```python
from build123d import *

# Parameters (mm, degrees)
SKETCH1_R           = 3.6
BOSS_EXTRUDE1_DEPTH = 14
BOSS_EXTRUDE2_DEPTH = 1.5
BOSS_EXTRUDE3_DEPTH = 9
CIRPATTERN1_COUNT   = 2


with BuildPart() as part:
    # Sketch1 → Boss-Extrude1 (new body)
    with BuildSketch(Plane(origin=(0, 0, 0), x_dir=(0, 0, -1), z_dir=(1, 0, 0))):
        Circle(SKETCH1_R)
    extrude(amount=BOSS_EXTRUDE1_DEPTH)

    # Sketch2 → Boss-Extrude2 (add)
    with BuildSketch(Plane.ZY):
        Polygon((-5, 16.642259954), (-3.505186232, 16.766886588), (-2.117676372, 0.124626634), (-3.61249014, 0), align=None)
    boss_extrude2 = extrude(amount=-BOSS_EXTRUDE2_DEPTH)

    # Sketch4 → Boss-Extrude3 (add)
    with BuildSketch(Plane(origin=(1.5, 0, 0), x_dir=(0, 0, -1), z_dir=(1, 0, 0))):
        Polygon((5, 16.642259954), (3.505186232, 16.766886588), (3.380559598, 15.27207282), (4.875373366, 15.147446186), align=None)
    boss_extrude3 = extrude(amount=BOSS_EXTRUDE3_DEPTH)

    # CirPattern1: Boss-Extrude2, Boss-Extrude3 ×2 about axis
    cirpattern1_axis = Axis((7, 0, 0), (0, 1, 0))
    add([boss_extrude2.rotate(cirpattern1_axis, i * 360 / CIRPATTERN1_COUNT) for i in range(1, CIRPATTERN1_COUNT)])
    add([boss_extrude3.rotate(cirpattern1_axis, i * 360 / CIRPATTERN1_COUNT) for i in range(1, CIRPATTERN1_COUNT)])


solid = part.part
```
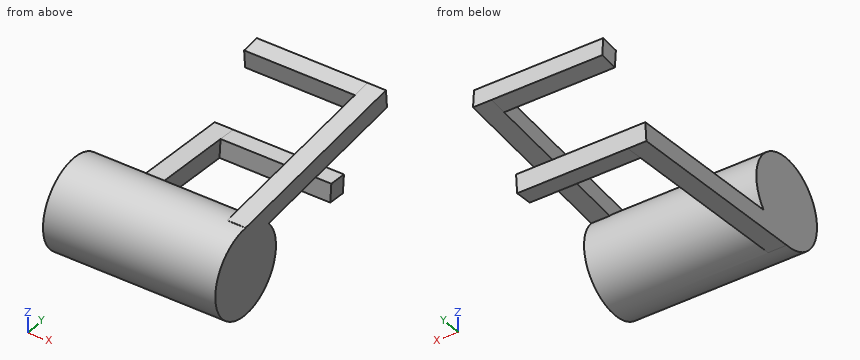
Geometry check sheet. Reference: the model listing, model coordinates, mm. Coordinates: 2 decimals unless noted, no trailing zeros. Write each loop counter-clockwise with the first axis right and the second up, starting at its lowest first coordinate (ties: lowest second). Pieces come first, ordered by that corner, then holes. Notation, with made-up numbers: M 16.5,83 L 44.5,83 A30 cw 44.5,107 Z; hole C 71,65 d5. An arc over 180 degrees is marked long. Use one line per item in the form item = value. Start each with the question number.
1) Thickness scan on probe 1 along Z at (x, y) = (2.5, 0); probe 2 along Z at (x, y) = (7.5, -2.5); probe 3 along Y at (x, z) = (9, 4.5). Record the ranges inside material, lowest first. Write a range as from..to.
2) Go/stop test with flat-tipped pins: pin 1 Ø3 at (y, z) = (7.5, -3.5) entering from +X; pin 2 Ø1.3 at (y, z) = (9.5, 4) entering from -X; pin 3 Ø4 at (x, y) = (5.5, 3.5) entering from +Z. Record where each tip stops, or that it passes through.
3) Section check D-D on y = 1.75. Enter the section's corners in (x, z), and give its area (3 significant figures).
4) Section check B-B on y = 9.75. Enter the section's corners in (x, z), and give its area (3 significant figures).
5) Section check C-C on x = 2.25. Enter the section's corners in (y, z), and give its area (3 significant figures).
6) Section check A-A on x = 8.5. Enter the section's corners in (y, z), and give its area (3 significant figures).
Responses:
q1.probe_1 = -3.6..3.6
q1.probe_2 = -2.59..2.59
q1.probe_3 = 15.18..16.68
q2.pin_1 = 1.5
q2.pin_2 = 12.5
q2.pin_3 = 3.27
q3.outline = M 0,-3.76 L 1.5,-3.76 L 1.5,-3.15 L 14,-3.15 L 14,3.76 L 12.5,3.76 L 12.5,3.15 L 0,3.15 Z
q3.area = 89.9 mm2
q4.outline = M 0,-4.43 L 1.5,-4.43 L 1.5,-2.92 L 0,-2.92 Z; M 12.5,2.92 L 14,2.92 L 14,4.43 L 12.5,4.43 Z
q4.area = 4.52 mm2
q5.outline = C 0,0 d7.2; M 15.15,-4.88 L 16.64,-5 L 16.77,-3.51 L 15.27,-3.38 Z
q5.area = 43.0 mm2
q6.outline = C 0,0 d7.2; M 15.15,-4.88 L 16.64,-5 L 16.77,-3.51 L 15.27,-3.38 Z; M 15.15,4.88 L 15.27,3.38 L 16.77,3.51 L 16.64,5 Z
q6.area = 45.2 mm2
